```python
from build123d import *

# Parameters (mm, degrees)
BOSS_EXTRUDE1_DEPTH = 25
SKETCH2_R           = 3.5
SKETCH2_R_2         = 1.5
CUT_EXTRUDE1_DEPTH  = 52.051444642
CIRPATTERN1_COUNT   = 3


with BuildPart() as part:
    # Sketch1 → Boss-Extrude1 (new, symmetric)
    with BuildSketch(Plane.XY):
        Polygon((22.5, -2.5), (-27.5, -2.5), (-27.5, 2.5), (22.5, 2.5), (22.5, 37.5), (27.5, 37.5), (27.5, -2.5), align=None)
    extrude(amount=BOSS_EXTRUDE1_DEPTH, both=True)

    # Sketch2 → Cut-Extrude1 (cut, through all)
    with BuildSketch(Plane(origin=(0, 2.5, 0), x_dir=(1, 0, 0), z_dir=(0, 1, 0))):
        with Locations(Location((0, 0, 0), (0, 0, 180))):
            Circle(SKETCH2_R)
        with Locations(Location((-3.623466631, 13.522961568, 0), (0, 0, 180))):
            Circle(SKETCH2_R_2)
        with Locations((3.623466631, 13.522961568)):
            Circle(SKETCH2_R_2)
    cut_extrude1 = extrude(amount=-CUT_EXTRUDE1_DEPTH, mode=Mode.SUBTRACT)

    # CirPattern1: Cut-Extrude1 ×3 about axis
    cirpattern1_axis = Axis((0, 0, 0), (0, 1, 0))
    for i in range(1, CIRPATTERN1_COUNT):
        add(cut_extrude1.rotate(cirpattern1_axis, i * 360 / CIRPATTERN1_COUNT), mode=Mode.SUBTRACT)


solid = part.part
```
CAD build for the part. Positions are in the model's coordinates, mm. A direction names the side the tool comes from. Round coordinates to 2 decimals unless told otherwise and drop trailing zeros. Order: outer loops, then holes, each group sorted by start corner. A loop starts at its lowest first (then second) coordinate and runs counter-clockwise, first axis right, second up.
Q1. Slice it at B-B (z = 0). Write the cut outline in (x, y).
Q2. Slice it at C-C (z = 6.5). Write the cut outline in (x, y), and give its area (3 significant figures).
Q3. Slice it at A-A (x = 0). Write the cut outline in (y, z), and give its area (3 significant figures).
Q4. Drop flat-ended pins along their axis: pin 1 (3 mm diameter, centred on x = 14, z = -14.5, fed in from +Y); pin 2 (10.5 mm diameter, centred on y = 22.5, z = 3, fed in from -X). Give the stop position or say it passes through.
Q5. Slice it at D-D (x = -20.5). Write the cut outline in (y, z), and give its area (3 significant figures).
Q6. Which spindle directions (+Z, -Z, +X, -X, +Y, -Y) get a long thin tool onto all of the face, cutting with end or side? Do faces 1 (the cylindrical face through (2.52, 0.04, -14.54)), 2 (the flat face through (22.5, 20, 0)). Say none if no direction does.
Q7. Wall check: L1, parallel to X at y = -1, z = 4.5; L2, parallel to Z at x = 0, y = 1; L3, parallel to Y at x = -8, z = 13. Give the ranges that are in metal, low to high.
Q8. Two-plate mould, pull along Z, no slides. Class faces 3 (the flat face through (12, 1, 25)), 4 (the cylindrical face through (-3.298, 0.035, -14.987)), 5 (the flat face through (25, 37.5, 0)): pulls with the +Z half, pulls with the -Z half, needs draft (parallel to the pull), parting line crosses it, or undercut.
Results below:
1. outline: (-27.5, -2.5) - (-3.5, -2.5) - (-3.5, 2.5) - (-27.5, 2.5) - close; (3.5, -2.5) - (27.5, -2.5) - (27.5, 37.5) - (22.5, 37.5) - (22.5, 2.5) - (3.5, 2.5) - close
2. outline: (-27.5, -2.5) - (27.5, -2.5) - (27.5, 37.5) - (22.5, 37.5) - (22.5, 2.5) - (-27.5, 2.5) - close
2. area: 450 mm2
3. outline: (-2.5, -25) - (2.5, -25) - (2.5, -3.5) - (-2.5, -3.5) - close; (-2.5, 3.5) - (2.5, 3.5) - (2.5, 25) - (-2.5, 25) - close
3. area: 215 mm2
4. pin 1: stops at y = 2.5
4. pin 2: stops at x = 22.5
5. outline: (-2.5, -25) - (2.5, -25) - (2.5, 25) - (-2.5, 25) - close
5. area: 250 mm2
6. face 1: +Y, -Y
6. face 2: +Z, -Z, -X, +Y
7. L1: x = -27.5 to -14.74, -12.31 to 12.31, 14.74 to 27.5
7. L2: z = -25 to -3.5, 3.5 to 25
7. L3: y = -2.5 to 2.5
8. face 3: pulls with the +Z half
8. face 4: undercut
8. face 5: needs draft
